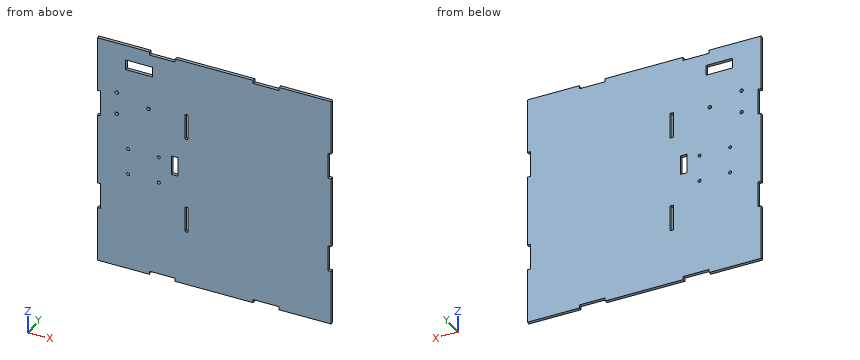
from build123d import *

# Parameters (mm, degrees)
SKETCH1_W           = 228.6
SKETCH1_H           = 228.6
BOSS_EXTRUDE1_DEPTH = 3.175
SKETCH2_R           = 1.7145
SKETCH2_R_2         = 1.5
SKETCH2_W           = 26
SKETCH2_H           = 10.000000066
SKETCH2_W_2         = 6.35
SKETCH2_H_2         = 19.05
CUT_EXTRUDE1_DEPTH  = 4.175
SKETCH3_W           = 3.175
SKETCH3_H           = 25.4
SKETCH3_W_2         = 25.4
SKETCH3_H_2         = 3.175
CUT_EXTRUDE2_DEPTH  = 4.175


with BuildPart() as part:
    # Sketch1 → Boss-Extrude1 (new body)
    with BuildSketch(Plane(origin=(0, 0, 0), x_dir=(1, 0, 0), z_dir=(0, 1, 0))):
        Rectangle(SKETCH1_W, SKETCH1_H)
    extrude(amount=BOSS_EXTRUDE1_DEPTH)

    # Sketch2 → Cut-Extrude1 (cut, through all)
    with BuildSketch(Plane(origin=(0, 3.175, 0), x_dir=(1, 0, 0), z_dir=(0, 1, 0))):
        with Locations((-95.250000001, -63.5)):
            Circle(SKETCH2_R)
        with Locations((-95.25, -41.5)):
            Circle(SKETCH2_R)
        with Locations((-64.250000001, -55.5)):
            Circle(SKETCH2_R)
        with Locations((-84.179457051, 17.330418354)):
            Circle(SKETCH2_R_2)
        with Locations((-54.207457051, 17.330418354)):
            Circle(SKETCH2_R_2)
        with Locations((-54.207457051, -8.577581646)):
            Circle(SKETCH2_R_2)
        with Locations((-84.179457051, -8.577581646)):
            Circle(SKETCH2_R_2)
        with Locations((-73.56649281, -94.479721333)):
            Rectangle(SKETCH2_W, SKETCH2_H)
        with Locations((-38.794244325, -4.118289102)):
            Rectangle(SKETCH2_W_2, SKETCH2_H_2)
    extrude(amount=-CUT_EXTRUDE1_DEPTH, mode=Mode.SUBTRACT)

    # Sketch3 → Cut-Extrude2 (cut, through all)
    with BuildSketch(Plane(origin=(0, 3.175, 0), x_dir=(1, 0, 0), z_dir=(0, 1, 0))):
        with Locations((-112.7125, 47.625)):
            Rectangle(SKETCH3_W, SKETCH3_H)
        with Locations((-112.7125, -47.625)):
            Rectangle(SKETCH3_W, SKETCH3_H)
        with Locations((112.7125, 47.625)):
            Rectangle(SKETCH3_W, SKETCH3_H)
        with Locations((112.7125, -47.625)):
            Rectangle(SKETCH3_W, SKETCH3_H)
        with Locations((50.8, -112.7125)):
            Rectangle(SKETCH3_W_2, SKETCH3_H_2)
        with Locations((-50.8, -112.7125)):
            Rectangle(SKETCH3_W_2, SKETCH3_H_2)
        with Locations((-50.8, 112.7125)):
            Rectangle(SKETCH3_W_2, SKETCH3_H_2)
        with Locations((50.8, 112.7125)):
            Rectangle(SKETCH3_W_2, SKETCH3_H_2)
        with Locations((-26.9875, -47.625)):
            Rectangle(SKETCH3_W, SKETCH3_H)
        with Locations((-26.9875, 47.625)):
            Rectangle(SKETCH3_W, SKETCH3_H)
    extrude(amount=-CUT_EXTRUDE2_DEPTH, mode=Mode.SUBTRACT)


solid = part.part
The model under review builds one solid part; all positions refer to its coordinate system, in mm. Give positions to 0.01 mm unless a question says otherwise; leave off trailing zeros. Write each loop counter-clockwise with the first axis right and the second up, starting at its lowest first coordinate (ties: lowest second). Pieces come first, ordered by that corner, then holes.
1. Add section A-A, the plane x = -70.5. Write out the cut boundary in (y, z) (3 decimals), plus the area to 3 significant figures.
2. For P1, Ø1, axis at x = -57, y = 3, coming from the +Z side (3 decimals); P2, Ø5, axis at x = -54.21, z = 8.58, coming from the +Y side (3 decimals), all flat-tipped, find the tip position at first contact; note any pin that passes through.
3. Wall thickness on L1, parallel to Z at x = -95.25, y = 2.5; L2, parallel to X at y = 2.7, z = 51 (3 decimals); L3, parallel to X at y = 1, z = 63.5: over which ranges is each line inside the solid? List them lowest first.
4. Add section B-B, the plane y = 2.4. Count the separate pieces of the cut face and the enclosed holes in it, plus the area to 3 significant figures.
Worked answers:
1. outline: (0, -114.3) - (3.175, -114.3) - (3.175, 89.48) - (0, 89.48) - close; (0, 99.48) - (3.175, 99.48) - (3.175, 114.3) - (0, 114.3) - close
1. area: 694 mm2
2. P1: stops at z = 111.125
2. P2: stops at y = 3.175
3. L1: z = -114.3 to 39.79, 43.21 to 61.79, 65.21 to 114.3
3. L2: x = -111.125 to -28.575, -25.4 to 111.125
3. L3: x = -114.3 to -96.96, -93.54 to 114.3
4. separate pieces: 1
4. enclosed holes: 11
4. area: 51,000 mm2
